```python
from build123d import *

# Parameters (mm, degrees)
SKETCH1_W           = 26
SKETCH1_H           = 19
BOSS_EXTRUDE1_DEPTH = 2
SKETCH2_W           = 12
SKETCH2_H           = 12
BOSS_EXTRUDE2_DEPTH = 7
SKETCH3_R           = 3.45
BOSS_EXTRUDE3_DEPTH = 7
SKETCH4_R           = 3.013235608
BOSS_EXTRUDE4_DEPTH = 13
CUT_EXTRUDE1_START  = -10
CUT_EXTRUDE1_DEPTH  = 10
FILLET1_R           = 0.4
SKETCH6_R           = 1.5
CUT_EXTRUDE2_DEPTH  = 43.023802843


with BuildPart() as part:
    # Sketch1 → Boss-Extrude1 (new body)
    with BuildSketch(Plane(origin=(0, 0, 0), x_dir=(1, 0, 0), z_dir=(0, 1, 0))):
        with Locations((13, 9.5)):
            Rectangle(SKETCH1_W, SKETCH1_H)
    extrude(amount=BOSS_EXTRUDE1_DEPTH)

    # Sketch2 → Boss-Extrude2 (add)
    with BuildSketch(Plane(origin=(0, 2, 0), x_dir=(1, 0, 0), z_dir=(0, 1, 0))):
        with Locations((15, 8)):
            Rectangle(SKETCH2_W, SKETCH2_H)
    extrude(amount=BOSS_EXTRUDE2_DEPTH)

    # Sketch3 → Boss-Extrude3 (add)
    with BuildSketch(Plane(origin=(0, 9, 0), x_dir=(1, 0, 0), z_dir=(0, 1, 0))):
        with Locations(Location((15, 8, 0), (0, 0, 270))):
            Circle(SKETCH3_R)
    extrude(amount=BOSS_EXTRUDE3_DEPTH)

    # Sketch4 → Boss-Extrude4 (add)
    with BuildSketch(Plane(origin=(0, 16, 0), x_dir=(1, 0, 0), z_dir=(0, 1, 0))):
        with Locations(Location((15, 8, 0), (0, 0, 90))):
            Circle(SKETCH4_R)
    extrude(amount=BOSS_EXTRUDE4_DEPTH)

    # Sketch5 → Cut-Extrude1 (cut)
    with BuildSketch(Plane(origin=(0, 29, 0), x_dir=(1, 0, 0), z_dir=(0, 1, 0)).offset(CUT_EXTRUDE1_START)):
        with BuildLine():
            Line((12.603290186, 9.826299784), (17.396709814, 9.826299784))
            ThreePointArc((17.396709814, 9.826299784), (15, 11.013235608), (12.603290186, 9.826299784))
        make_face()
    extrude(amount=CUT_EXTRUDE1_DEPTH, mode=Mode.SUBTRACT)

    # Fillet1
    fillet1_edges = [part.edges().sort_by_distance(p)[0] for p in [
        (15, 29, -4.986764392),
    ]]
    fillet(fillet1_edges, radius=FILLET1_R)

    # Sketch6 → Cut-Extrude2 (cut, through all)
    with BuildSketch(Plane(origin=(0, 2, 0), x_dir=(1, 0, 0), z_dir=(0, 1, 0))):
        with Locations(Location((21.5, 16, 0), (0, 0, 270))):
            Circle(SKETCH6_R)
        with Locations(Location((4.5, 16, 0), (0, 0, 270))):
            Circle(SKETCH6_R)
    extrude(amount=-CUT_EXTRUDE2_DEPTH, mode=Mode.SUBTRACT)


solid = part.part
```
For this review, take the finished solid that the model builds, in its own axes (mm). A direction names the side the tool comes from. Round coordinates to 2 decimals unless told otherwise and drop trailing zeros. Order: outer loops, then holes, each group sorted by start corner. A loop starts at its lowest first (then second) coordinate and runs counter-clockwise, first axis right, second up. Notation, with made-up numbers: (5.25, 4) -> (50.25, 4) arc R24 cw to (50.25, 21) -> close; hole circle Ø9 at (42, 14). An arc over 180 degrees is marked (long way). Use a Markdown table: item, result.
Item 1: Take a section at D-D (y = 23.25). State the section outline as (x, z) points.
Resolved:
| item | result |
|---|---|
| outline | (12.6, -9.83) -> (17.4, -9.83) arc R3.01 ccw (long way) to start |
Item 2: For line 1 along X through (y, z) = (1.55, -16); line 2 along Y through (x, z) = (8.75, -1.25); line 3 along Y through (x, z) = (12.25, -11), list the stretches that pass through material, from the lowest coordinate up. Write a range as [from, to].
Resolved:
| item | result |
|---|---|
| line 1 | x = [0, 3], [6, 20], [23, 26] |
| line 2 | y = [0, 2] |
| line 3 | y = [0, 9] |
Item 3: Take a section at C-C (x = 15). State the section outline as (y, z) points, plus the area to 3 significant figures.
Resolved:
| item | result |
|---|---|
| outline | (0, -19) -> (2, -19) -> (2, -14) -> (9, -14) -> (9, -11.45) -> (16, -11.45) -> (16, -11.01) -> (19, -11.01) -> (19, -9.83) -> (29, -9.83) -> (29, -5.39) arc R0.4 ccw to (28.6, -4.99) -> (16, -4.99) -> (16, -4.55) -> (9, -4.55) -> (9, -2) -> (2, -2) -> (2, 0) -> (0, 0) -> close |
| area | 237 mm² |
Item 4: Draft analysis for pull direction X (two halves, no side actions). For faces 5 (the cylindrical face through (22.51, 1.01, -17.11)), 6 (the flat face through (9, 5, -8)), 7 (the flat face through (13, 1, 0)), 8 (the cylindrical face through (18.42, 12.45, -8.45)), state which applies: +X half, -X half, draft (parallel to the pull), parting line (faces both ways), or undercut.
Resolved:
| item | result |
|---|---|
| face 5 | undercut |
| face 6 | -X half |
| face 7 | draft |
| face 8 | parting line |
Item 5: Take a section at B-B (z = -8). State the section outline as (x, y) points, plus the area to 3 significant figures.
Resolved:
| item | result |
|---|---|
| outline | (0, 0) -> (26, 0) -> (26, 2) -> (21, 2) -> (21, 9) -> (18.45, 9) -> (18.45, 16) -> (18.01, 16) -> (18.01, 28.6) arc R0.4 ccw to (17.61, 29) -> (12.39, 29) arc R0.4 ccw to (11.99, 28.6) -> (11.99, 16) -> (11.55, 16) -> (11.55, 9) -> (9, 9) -> (9, 2) -> (0, 2) -> close |
| area | 263 mm² |
Item 6: Take a section at A-A (x = 21.5). State the section outline as (y, z) points.
Resolved:
| item | result |
|---|---|
| outline | (0, -19) -> (2, -19) -> (2, -17.5) -> (0, -17.5) -> close; (0, -14.5) -> (2, -14.5) -> (2, 0) -> (0, 0) -> close |
Item 7: For pin 1 (2 mm diameter, centred on x = 13, y = 6, fed in from -Z); pin 2 (5 mm diameter, centred on y = 18.5, z = -11, fed in from -X); pin 3 (3.5 mm diameter, centred on x = 16.5, y = 5.5, fed in from +Z), all flat-tipped, find the tip position at first contact; note any pin that passes through.
Resolved:
| item | result |
|---|---|
| pin 1 | stops at z = -14 |
| pin 2 | stops at x = 12.03 |
| pin 3 | stops at z = -2 |
Item 8: Machinability: for faces 1 (the flat face through (18, 9, -11)), 2 (the flat face through (15, 19, -10)), 3 (the flat face through (15, 5, -2)), 4 (the flat face through (21, 5, -8)), which of the approach directions +Z, -Z, +X, -X, +Y, -Y give a long, thin tool a straight path to every point of the face, cutting with its end or side? Answer none if there is none.
Resolved:
| item | result |
|---|---|
| face 1 | +Y |
| face 2 | -Z, +X, -X, +Y |
| face 3 | +Z, +X, -X, +Y |
| face 4 | +Z, -Z, +X, +Y |
